```python
from build123d import *

# Parameters (mm, degrees)
F1_DEPTH = 19.05
F0_W     = 50.8
F0_H     = 44.45
F2_DEPTH = 44.45
F3_SIZE  = 12.7
F5_D     = 25.4


with BuildPart() as f1:
    # F0 (on Top) → F1 (new body)
    with BuildSketch(Plane.XY):
        Polygon((-26.007392, 0), (-6.957392, 0), (-6.957392, 16.002), (5.742608, 16.002), (5.742608, 0), (24.792608, 0), (24.792608, 31.75), (-26.007392, 31.75), align=None)
    extrude(amount=F1_DEPTH)

    # F0 (on Top) → F2 (join)
    with BuildSketch(Plane.XY):
        with Locations((-0.607392, 53.975)):
            Rectangle(F0_W, F0_H)
    extrude(amount=F2_DEPTH)

    # F3
    f3_edges = [f1.edges().sort_by_distance(p)[0] for p in [
        (24.792608, 76.2, 22.225),
        (-26.007392, 76.2, 22.225),
    ]]
    chamfer(f3_edges, length=F3_SIZE)

    # F5 (through all)
    with Locations(Plane.XY.offset(44.45)):
        with Locations((-0.607392, 53.848)):
            Hole(F5_D / 2)


solid = f1.part
```
Geometry check sheet. Reference: the model listing, model coordinates, mm. A direction names the side the tool comes from. Round coordinates to 2 decimals unless told otherwise and drop trailing zeros. Order: outer loops, then holes, each group sorted by start corner. A loop starts at its lowest first (then second) coordinate and runs counter-clockwise, first axis right, second up. Notation, with made-up numbers: M -15.5,-36 L -4.5,-36 A23 cw -4.5,-3 Z; hole C 46,-12 d9. An arc over 180 degrees is marked long. Answer as CSV lines item,"result".
1) Gauge pin test, flat ends, axial feed: pin 1 Ø1.5 at (x, z) = (16.5, 32.5) entering from +Y; pin 2 Ø10 at (x, z) = (-1.5, 8) entering from -Y; pin 3 Ø5 at (x, y) = (11.5, 10) entering from +Z. Record the tip position at first contact, or that the pin passes through.
Entries:
pin 1,"y = 72.54"
pin 2,"y = 16"
pin 3,"z = 19.05"
2) Sectioned sample at B-B on z = 23. Record the cut outline in (x, y).
Entries:
outline,"M -26.01,31.75 L 24.79,31.75 L 24.79,63.5 L 12.09,76.2 L -13.31,76.2 L -26.01,63.5 Z; hole C -0.61,53.85 d25.4"
3) Mould release check, pull along X, two halves, no side actions. Record for faces 4 (the face through (15, 0, 9)), 5 (the face through (18.35, 69.94, 21.91)), 6 (the face through (1.05, 66.44, 21.91)): +X half, -X half, draft (parallel to the pull), parting line (faces both ways), or undercut.
Entries:
face 4,"draft"
face 5,"+X half"
face 6,"undercut"
4) Thickness scan on probe 1 along Z at (x, y) = (18, 11); probe 2 along X at (y, z) = (43.5, 42.5); probe 3 along X at (y, z) = (45.5, 33.5). Record the ranges inside material, lowest first. Write a range as [from, to].
Entries:
probe 1,"[0, 19.05]"
probe 2,"[-26.01, -7.97], [6.76, 24.79]"
probe 3,"[-26.01, -10.18], [8.96, 24.79]"
5) Sectioned sample at A-A on y = 62. Record the cut outline in (x, z), and give its area (3 significant figures).
Entries:
outline,"M -26.01,0 L -10.35,0 L -10.35,44.45 L -26.01,44.45 Z; M 9.13,0 L 24.79,0 L 24.79,44.45 L 9.13,44.45 Z"
area,"1,390 mm2"
6) Sectioned sample at D-D on y = 49. Record the cut outline in (x, z).
Entries:
outline,"M -26.01,0 L -12.35,0 L -12.35,44.45 L -26.01,44.45 Z; M 11.13,0 L 24.79,0 L 24.79,44.45 L 11.13,44.45 Z"
7) Sectioned sample at C-C on x = 15. Record the cut outline in (y, z).
Entries:
outline,"M 0,0 L 73.29,0 L 73.29,44.45 L 31.75,44.45 L 31.75,19.05 L 0,19.05 Z"
8) Tool access check on faces 1 (the face through (-1, 20, 19.05)), 2 (the face through (5.743, 8, 9)), 3 (the face through (-1, 39, 44.45)). Record the directions out of +Z, -Z, +X, -X, +Y, -Y that give a thin tool (end or side, any length) a straight path to the whole face; none if there is none.
Entries:
face 1,"+Z, +X, -X, -Y"
face 2,"+Z, -Z, -Y"
face 3,"+Z, +X, -X, +Y, -Y"
